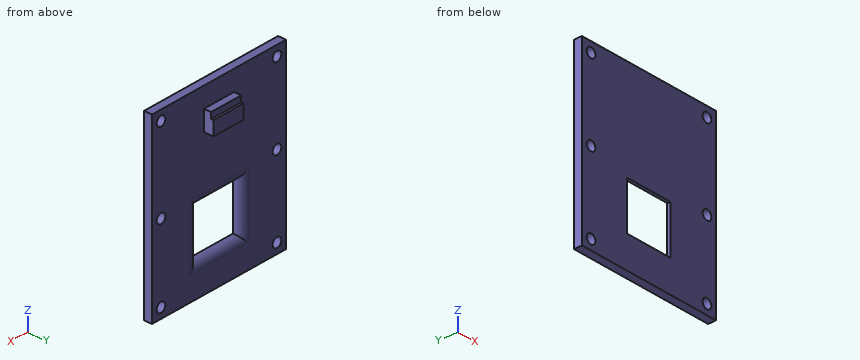
```python
from build123d import *

# Parameters (mm, degrees)
SKETCH1_W            = 27
SKETCH1_H            = 35
SKETCH1_R            = 1.113712744
SKETCH1_R_2          = 1.000106258
SKETCH1_R_3          = 1.174626552
SKETCH1_R_4          = 1.19920455
SKETCH1_W_2          = 8.3
SKETCH1_H_2          = 2.12
BOSS_EXTRUDE1_DEPTH  = 2
CUT_EXTRUDE2_REACH   = 25.536
SKETCH10_W           = 12
SKETCH10_H           = 12
FILLET1_R            = 2
SKETCH12_W           = 8.3
SKETCH12_H           = 1.5
BOSS_EXTRUDE5_DEPTH  = 1.8
SKETCH13_W           = 8.3
SKETCH13_H           = 3.507295064
BOSS_EXTRUDE6_DEPTH  = 2.395619389
SKETCH14_W           = 37
SKETCH14_H           = 45
SKETCH14_W_2         = 27
SKETCH14_H_2         = 35
BOSS_EXTRUDE7_DEPTH  = 2
M2_CLEARANCE_HOLE3_D = 2.4


with BuildPart() as part:
    # Sketch1 → Boss-Extrude1 (new body)
    # profile 1 of 8: a face of its own
    with BuildSketch(Plane(origin=(0, 0, 0), x_dir=(1, 0, 0), z_dir=(0, 1, 0))):
        with Locations((0.988085162, -0.939800033)):
            Rectangle(SKETCH1_W, SKETCH1_H)
        Polygon((-10.011914838, -15.939800033), (-10.011914838, 14.060199967), (11.988085162, 14.060199967), (11.988085162, -15.939800033), (5.138085162, -15.939800033), (5.138085162, -18.059800033), (-3.161914838, -18.059800033), (-3.161914838, -15.939800033), align=None, mode=Mode.SUBTRACT)
    # profile 2 of 8: a face of its own
    with BuildSketch(Plane(origin=(0, 0, 0), x_dir=(1, 0, 0), z_dir=(0, 1, 0))):
        Polygon((11.988085162, 14.060199967), (-10.011914838, 14.060199967), (-10.011914838, -15.939800033), (-3.161914838, -15.939800033), (-3.161914838, -13.819800033), (5.138085162, -13.819800033), (5.138085162, -15.939800033), (11.988085162, -15.939800033), align=None)
        with Locations((-8.011914838, -13.939800033)):
            Circle(SKETCH1_R, mode=Mode.SUBTRACT)
        with Locations((9.988085162, -14.291814947)):
            Circle(SKETCH1_R_2, mode=Mode.SUBTRACT)
        with Locations((-8.011914838, 7.560199967)):
            Circle(SKETCH1_R_3, mode=Mode.SUBTRACT)
        with Locations((9.988085162, 7.560199967)):
            Circle(SKETCH1_R_4, mode=Mode.SUBTRACT)
    # profile 3 of 8: a face of its own
    with BuildSketch(Plane(origin=(0, 0, 0), x_dir=(1, 0, 0), z_dir=(0, 1, 0))):
        with Locations((-8.011914838, 7.560199967)):
            Circle(SKETCH1_R_3)
    # profile 4 of 8: a face of its own
    with BuildSketch(Plane(origin=(0, 0, 0), x_dir=(1, 0, 0), z_dir=(0, 1, 0))):
        with Locations((9.988085162, 7.560199967)):
            Circle(SKETCH1_R_4)
    # profile 5 of 8: a face of its own
    with BuildSketch(Plane(origin=(0, 0, 0), x_dir=(1, 0, 0), z_dir=(0, 1, 0))):
        with Locations((9.988085162, -14.291814947)):
            Circle(SKETCH1_R_2)
    # profile 6 of 8: a face of its own
    with BuildSketch(Plane(origin=(0, 0, 0), x_dir=(1, 0, 0), z_dir=(0, 1, 0))):
        with Locations((0.988085162, -16.999800033)):
            Rectangle(SKETCH1_W_2, SKETCH1_H_2)
    # profile 7 of 8: a face of its own
    with BuildSketch(Plane(origin=(0, 0, 0), x_dir=(1, 0, 0), z_dir=(0, 1, 0))):
        with Locations((0.988085162, -14.879800033)):
            Rectangle(SKETCH1_W_2, SKETCH1_H_2)
    # profile 8 of 8: a face of its own
    with BuildSketch(Plane(origin=(0, 0, 0), x_dir=(1, 0, 0), z_dir=(0, 1, 0))):
        with Locations((-8.011914838, -13.939800033)):
            Circle(SKETCH1_R)
    extrude(amount=BOSS_EXTRUDE1_DEPTH)

    # Sketch10 → Cut-Extrude2 (cut, up to next)
    with BuildSketch(Plane(origin=(0, 2, 0), x_dir=(1, 0, 0), z_dir=(0, 1, 0)), mode=Mode.PRIVATE) as cut_extrude2_sk1:
        with Locations((0.938085162, 7.590199967)):
            Rectangle(SKETCH10_W, SKETCH10_H)
    cut_extrude2_tool1 = extrude(cut_extrude2_sk1.sketch, amount=-CUT_EXTRUDE2_REACH, mode=Mode.PRIVATE) & part.part
    add(cut_extrude2_tool1.solids().sort_by_distance((0.938085, 2, -7.5902))[0], mode=Mode.SUBTRACT)

    # Fillet1
    fillet1_edges = [part.edges().sort_by_distance(p)[0] for p in [
        (0.938085162, 2, -13.590199967),
        (6.938085162, 2, -7.590199967),
        (0.938085162, 2, -1.590199967),
        (-5.061914838, 2, -7.590199967),
    ]]
    fillet(fillet1_edges, radius=FILLET1_R - 0.0001)  # a hair under: the kernel refuses the full size

    # Sketch12 → Boss-Extrude5 (add)
    with BuildSketch(Plane(origin=(0, 2, 0), x_dir=(1, 0, 0), z_dir=(0, 1, 0))):
        with Locations((0.988085162, -17.689800033)):
            Rectangle(SKETCH12_W, SKETCH12_H)
    extrude(amount=BOSS_EXTRUDE5_DEPTH)

    # Sketch13 → Boss-Extrude6 (add)
    with BuildSketch(Plane(origin=(0, 2, 0), x_dir=(1, 0, 0), z_dir=(0, 1, 0))):
        with Locations((0.988085162, -15.186152501)):
            Rectangle(SKETCH13_W, SKETCH13_H)
    extrude(amount=BOSS_EXTRUDE6_DEPTH)

    # Sketch14 → Boss-Extrude7 (add)
    with BuildSketch(Plane.XZ):
        with Locations((0.988085162, 0.939800033)):
            Rectangle(SKETCH14_W, SKETCH14_H)
        with Locations((0.988085162, 0.939800033)):
            Rectangle(SKETCH14_W_2, SKETCH14_H_2, mode=Mode.SUBTRACT)
    extrude(amount=-BOSS_EXTRUDE7_DEPTH)

    # M2 Clearance Hole3 (through all)
    with Locations(Plane(origin=(0, 0, 0), x_dir=(-1, 0, 0), z_dir=(0, -1, 0))):
        with Locations((-16.988085162, 19.060199967), (15.011914838, 19.060199967), (15.011914838, -0.939800033), (15.011914838, -20.939800033), (-16.988085162, -20.939800033), (-16.988085162, -1.8e-07)):
            Hole(M2_CLEARANCE_HOLE3_D / 2)


solid = part.part
```
Part model, mm, in its own coordinate system. Round coordinates to 2 decimals unless told otherwise and drop trailing zeros. Loops run counter-clockwise (first coordinate to the right, second up) from the corner with the lowest first, then second, coordinate; pieces in that order, holes last.
Item 1: Cut at B-B, the plane x = -15. Give the cut face in (y, z), then the cut area to 3 significant figures.
Item 2: Drill centre lines: line 1 (Y direction, x = -10.5, z = -1); line 2 (X direction, y = 1.3, z = -10); line 3 (Z direction, x = -4, y = 1.15). Where is each one in solid material? Low to high.
Item 3: Drop flat-ended pins along their axis: P1, Ø3, axis at x = -15.01, z = 0.94, coming from the +Y side; P2, Ø1.9, axis at y = 3.5, z = 15.5, coming from the -X side; P3, Ø1.2, axis at x = 0, y = 3, coming from the -Z side. Give the stop position or say it passes through.
Item 4: Cut at C-C, the plane y = 0.95. Give the cut face in (x, z).
Item 5: Cut at D-D, the plane z = 11.5. Give the cut face in (x, y).
A:
1. outline: (0, -21.56) - (2, -21.56) - (2, -20.26) - (0, -20.26) - close; (0, -17.86) - (2, -17.86) - (2, -0.26) - (0, -0.26) - close; (0, 2.14) - (2, 2.14) - (2, 19.74) - (0, 19.74) - close; (0, 22.14) - (2, 22.14) - (2, 23.44) - (0, 23.44) - close
1. area: 75.6 mm2
2. line 1: y = 0 to 2
2. line 2: x = -17.51 to -5.54, 7.42 to 19.49
2. line 3: z = -21.56 to -13.95, -1.23 to 23.44
3. P1: stops at y = 2
3. P2: stops at x = -3.16
3. P3: stops at z = 13.43
4. outline: (-17.51, -21.56) - (19.49, -21.56) - (19.49, 23.44) - (-17.51, 23.44) - close; hole circle Ø2.4 at (-15.01, -19.06); hole circle Ø2.4 at (-15.01, 0.94); hole circle Ø2.4 at (-15.01, 20.94); hole (-5.3, -13.83) - (7.18, -13.83) - (7.18, -1.35) - (-5.3, -1.35) - close; hole circle Ø2.4 at (16.99, -19.06); hole circle Ø2.4 at (16.99, 0); hole circle Ø2.4 at (16.99, 20.94)
5. outline: (-17.51, 0) - (19.49, 0) - (19.49, 2) - (-17.51, 2) - close
